The model under review builds one solid part; all positions refer to its coordinate system, in mm. A direction names the side the tool comes from. Round coordinates to 2 decimals unless told otherwise and drop trailing zeros. Order: outer loops, then holes, each group sorted by start corner. A loop starts at its lowest first (then second) coordinate and runs counter-clockwise, first axis right, second up.
```python
from build123d import *

# Parameters (mm, degrees)
SKETCH1_W           = 96.799999948
SKETCH1_H           = 98
BOSS_EXTRUDE1_DEPTH = 1.2192
CUT_EXTRUDE1_REACH  = 139.752
SKETCH5_R           = 1.0922
CUT_EXTRUDE2_REACH  = 139.752
SKETCH6_R           = 1.143
SKETCH10_W          = 5
SKETCH10_H          = 5.08
SKETCH10_R          = 1.143
BOSS_EXTRUDE2_DEPTH = 96.774
SKETCH13_W          = 86.614
SKETCH13_H          = 5
CUT_EXTRUDE3_DEPTH  = 5.08
BOSS_EXTRUDE3_DEPTH = 5.08
BOSS_EXTRUDE5_DEPTH = 5.08
BOSS_EXTRUDE6_DEPTH = 5.08
BOSS_EXTRUDE7_DEPTH = 5.08
BOSS_EXTRUDE8_DEPTH = 5.08


with BuildPart() as part:
    # Sketch1 → Boss-Extrude1 (new body)
    with BuildSketch(Plane(origin=(0, 0, 0), x_dir=(1, 0, 0), z_dir=(0, 1, 0))):
        with Locations((48.399999974, -49)):
            Rectangle(SKETCH1_W, SKETCH1_H)
    extrude(amount=BOSS_EXTRUDE1_DEPTH)

    # Sketch5 → Cut-Extrude1 (cut, up to next)
    with BuildSketch(Plane(origin=(0, 0, 0), x_dir=(-1, 0, 0), z_dir=(0, -1, 0)), mode=Mode.PRIVATE) as cut_extrude1_sk1:
        with Locations(Location((-3.5, -94.5, 0), (0, 0, 90))):
            Circle(SKETCH5_R)
    cut_extrude1_tool1 = extrude(cut_extrude1_sk1.sketch, amount=-CUT_EXTRUDE1_REACH, mode=Mode.PRIVATE) & part.part
    # Sketch5 → Cut-Extrude1 (cut, up to next)
    with BuildSketch(Plane(origin=(0, 0, 0), x_dir=(-1, 0, 0), z_dir=(0, -1, 0)), mode=Mode.PRIVATE) as cut_extrude1_sk2:
        with Locations(Location((-7.7, -95.3, 0), (0, 0, 90))):
            Circle(SKETCH5_R)
    cut_extrude1_tool2 = extrude(cut_extrude1_sk2.sketch, amount=-CUT_EXTRUDE1_REACH, mode=Mode.PRIVATE) & part.part
    # Sketch5 → Cut-Extrude1 (cut, up to next)
    with BuildSketch(Plane(origin=(0, 0, 0), x_dir=(-1, 0, 0), z_dir=(0, -1, 0)), mode=Mode.PRIVATE) as cut_extrude1_sk3:
        with Locations(Location((-21.3, -95.3, 0), (0, 0, 90))):
            Circle(SKETCH5_R)
    cut_extrude1_tool3 = extrude(cut_extrude1_sk3.sketch, amount=-CUT_EXTRUDE1_REACH, mode=Mode.PRIVATE) & part.part
    # Sketch5 → Cut-Extrude1 (cut, up to next)
    with BuildSketch(Plane(origin=(0, 0, 0), x_dir=(-1, 0, 0), z_dir=(0, -1, 0)), mode=Mode.PRIVATE) as cut_extrude1_sk4:
        with Locations(Location((-93.3, -94.5, 0), (0, 0, 90))):
            Circle(SKETCH5_R)
    cut_extrude1_tool4 = extrude(cut_extrude1_sk4.sketch, amount=-CUT_EXTRUDE1_REACH, mode=Mode.PRIVATE) & part.part
    # Sketch5 → Cut-Extrude1 (cut, up to next)
    with BuildSketch(Plane(origin=(0, 0, 0), x_dir=(-1, 0, 0), z_dir=(0, -1, 0)), mode=Mode.PRIVATE) as cut_extrude1_sk5:
        with Locations(Location((-93.3, -16.5, 0), (0, 0, 90))):
            Circle(SKETCH5_R)
    cut_extrude1_tool5 = extrude(cut_extrude1_sk5.sketch, amount=-CUT_EXTRUDE1_REACH, mode=Mode.PRIVATE) & part.part
    # Sketch5 → Cut-Extrude1 (cut, up to next)
    with BuildSketch(Plane(origin=(0, 0, 0), x_dir=(-1, 0, 0), z_dir=(0, -1, 0)), mode=Mode.PRIVATE) as cut_extrude1_sk6:
        with Locations(Location((-3.5, -16.5, 0), (0, 0, 90))):
            Circle(SKETCH5_R)
    cut_extrude1_tool6 = extrude(cut_extrude1_sk6.sketch, amount=-CUT_EXTRUDE1_REACH, mode=Mode.PRIVATE) & part.part
    # Sketch5 → Cut-Extrude1 (cut, up to next)
    with BuildSketch(Plane(origin=(0, 0, 0), x_dir=(-1, 0, 0), z_dir=(0, -1, 0)), mode=Mode.PRIVATE) as cut_extrude1_sk7:
        with Locations(Location((-7.7, -15.7, 0), (0, 0, 90))):
            Circle(SKETCH5_R)
    cut_extrude1_tool7 = extrude(cut_extrude1_sk7.sketch, amount=-CUT_EXTRUDE1_REACH, mode=Mode.PRIVATE) & part.part
    # Sketch5 → Cut-Extrude1 (cut, up to next)
    with BuildSketch(Plane(origin=(0, 0, 0), x_dir=(-1, 0, 0), z_dir=(0, -1, 0)), mode=Mode.PRIVATE) as cut_extrude1_sk8:
        with Locations(Location((-21.3, -15.7, 0), (0, 0, 90))):
            Circle(SKETCH5_R)
    cut_extrude1_tool8 = extrude(cut_extrude1_sk8.sketch, amount=-CUT_EXTRUDE1_REACH, mode=Mode.PRIVATE) & part.part
    add(cut_extrude1_tool1.solids().sort_by_distance((3.5, 0, 94.5))[0], mode=Mode.SUBTRACT)
    add(cut_extrude1_tool2.solids().sort_by_distance((7.7, 0, 95.3))[0], mode=Mode.SUBTRACT)
    add(cut_extrude1_tool3.solids().sort_by_distance((21.3, 0, 95.3))[0], mode=Mode.SUBTRACT)
    add(cut_extrude1_tool4.solids().sort_by_distance((93.3, 0, 94.5))[0], mode=Mode.SUBTRACT)
    add(cut_extrude1_tool5.solids().sort_by_distance((93.3, 0, 16.5))[0], mode=Mode.SUBTRACT)
    add(cut_extrude1_tool6.solids().sort_by_distance((3.5, 0, 16.5))[0], mode=Mode.SUBTRACT)
    add(cut_extrude1_tool7.solids().sort_by_distance((7.7, 0, 15.7))[0], mode=Mode.SUBTRACT)
    add(cut_extrude1_tool8.solids().sort_by_distance((21.3, 0, 15.7))[0], mode=Mode.SUBTRACT)

    # Sketch6 → Cut-Extrude2 (cut, up to next)
    with BuildSketch(Plane(origin=(0, 1.2192, 0), x_dir=(1, 0, 0), z_dir=(0, 1, 0)), mode=Mode.PRIVATE) as cut_extrude2_sk1:
        with Locations(Location((56.337499948, -7.540625, 0), (0, 0, 270))):
            Circle(SKETCH6_R)
    cut_extrude2_tool1 = extrude(cut_extrude2_sk1.sketch, amount=-CUT_EXTRUDE2_REACH, mode=Mode.PRIVATE) & part.part
    # Sketch6 → Cut-Extrude2 (cut, up to next)
    with BuildSketch(Plane(origin=(0, 1.2192, 0), x_dir=(1, 0, 0), z_dir=(0, 1, 0)), mode=Mode.PRIVATE) as cut_extrude2_sk2:
        with Locations(Location((40.462499948, -7.540625, 0), (0, 0, 270))):
            Circle(SKETCH6_R)
    cut_extrude2_tool2 = extrude(cut_extrude2_sk2.sketch, amount=-CUT_EXTRUDE2_REACH, mode=Mode.PRIVATE) & part.part
    # Sketch6 → Cut-Extrude2 (cut, up to next)
    with BuildSketch(Plane(origin=(0, 1.2192, 0), x_dir=(1, 0, 0), z_dir=(0, 1, 0)), mode=Mode.PRIVATE) as cut_extrude2_sk3:
        with Locations(Location((40.462499948, -90.459375, 0), (0, 0, 270))):
            Circle(SKETCH6_R)
    cut_extrude2_tool3 = extrude(cut_extrude2_sk3.sketch, amount=-CUT_EXTRUDE2_REACH, mode=Mode.PRIVATE) & part.part
    # Sketch6 → Cut-Extrude2 (cut, up to next)
    with BuildSketch(Plane(origin=(0, 1.2192, 0), x_dir=(1, 0, 0), z_dir=(0, 1, 0)), mode=Mode.PRIVATE) as cut_extrude2_sk4:
        with Locations(Location((56.337499948, -90.459375, 0), (0, 0, 270))):
            Circle(SKETCH6_R)
    cut_extrude2_tool4 = extrude(cut_extrude2_sk4.sketch, amount=-CUT_EXTRUDE2_REACH, mode=Mode.PRIVATE) & part.part
    add(cut_extrude2_tool1.solids().sort_by_distance((56.3375, 1.2192, 7.540625))[0], mode=Mode.SUBTRACT)
    add(cut_extrude2_tool2.solids().sort_by_distance((40.4625, 1.2192, 7.540625))[0], mode=Mode.SUBTRACT)
    add(cut_extrude2_tool3.solids().sort_by_distance((40.4625, 1.2192, 90.459375))[0], mode=Mode.SUBTRACT)
    add(cut_extrude2_tool4.solids().sort_by_distance((56.3375, 1.2192, 90.459375))[0], mode=Mode.SUBTRACT)

    # Sketch10 → Boss-Extrude2 (add)
    with BuildSketch(Plane(origin=(96.799999948, 0, 0), x_dir=(0, 0, -1), z_dir=(1, 0, 0))):
        with Locations((-49, 3.7592)):
            Rectangle(SKETCH10_W, SKETCH10_H)
        with Locations((-49, 2.64795)):
            Circle(SKETCH10_R, mode=Mode.SUBTRACT)
    extrude(amount=-BOSS_EXTRUDE2_DEPTH)

    # Sketch13 → Cut-Extrude3 (cut)
    with BuildSketch(Plane(origin=(0, 6.2992, 0), x_dir=(1, 0, 0), z_dir=(0, 1, 0))):
        with Locations((48.412999948, -49)):
            Rectangle(SKETCH13_W, SKETCH13_H)
    extrude(amount=-CUT_EXTRUDE3_DEPTH, mode=Mode.SUBTRACT)

    # Sketch14 → Boss-Extrude3 (add)
    with BuildSketch(Plane.XZ):
        Polygon((0, 49), (0, 51.54), (5.08, 51.54), (5.08, 46.46), (0, 46.46), align=None)
        Polygon((96.799999948, 49), (96.799999948, 51.54), (91.719999948, 51.54), (91.719999948, 46.46), (96.799999948, 46.46), align=None)
    extrude(amount=BOSS_EXTRUDE3_DEPTH)

    # Sketch15 → Boss-Extrude5 (add)
    with BuildSketch(Plane.ZY):
        Polygon((51.54, -5.08), (46.46, -5.08), (46.46, -5.479804671), align=None)
    extrude(amount=-BOSS_EXTRUDE5_DEPTH)

    # Sketch16 → Boss-Extrude6 (add)
    with BuildSketch(Plane(origin=(96.799999948, 0, 0), x_dir=(0, 0, -1), z_dir=(1, 0, 0))):
        Polygon((-46.46, -5.08), (-51.54, -5.08), (-46.46, -5.479804671), align=None)
    extrude(amount=-BOSS_EXTRUDE6_DEPTH)

    # Sketch17 → Boss-Extrude7 (add)
    with BuildSketch(Plane(origin=(96.799999948, 0, 0), x_dir=(0, 0, -1), z_dir=(1, 0, 0))):
        Polygon((-46.5, 6.2992), (-51.5, 6.2992), (-51.5, 6.692708534), align=None)
    extrude(amount=-BOSS_EXTRUDE7_DEPTH)

    # Sketch18 → Boss-Extrude8 (add)
    with BuildSketch(Plane.ZY.offset(-0.025999948)):
        Polygon((46.5, 6.2992), (51.5, 6.2992), (51.5, 6.692708534), align=None)
    extrude(amount=-BOSS_EXTRUDE8_DEPTH)


solid = part.part
```
(1) Consider section A-A (y = -2). Write out the cut boundary in (x, z), and give its area (3 significant figures).
Data:
outline: (0, 46.46) - (5.08, 46.46) - (5.08, 51.54) - (0, 51.54) - close; (91.72, 46.46) - (96.8, 46.46) - (96.8, 51.54) - (91.72, 51.54) - close
area: 51.6 mm2
(2) To check wall thickness, follow probe 1 along Z at (x, y) = (93.3, 0.7); probe 2 along X at (y, z) = (0.9, 94.5); probe 3 along Y at (x, z) = (58, 84). State the ranges of each line that lie inside material, in increasing order.
Data:
probe 1: z = 0 to 15.41, 17.59 to 93.41, 95.59 to 98
probe 2: x = 0 to 2.41, 4.59 to 6.96, 8.44 to 20.56, 22.04 to 92.21, 94.39 to 96.8
probe 3: y = 0 to 1.22
(3) Insertion check: pin 1 (1.7 mm diameter, centred on x = 3.5, z = 16.5, fed in from -Y); pin 2 (1.5 mm diameter, centred on x = 2.5, y = 3.5, fed in from +Z); pin 3 (3 mm diameter, centred on x = 40.46, z = 90.46, fed in from -Y); pin 4 (4 mm diameter, centred on x = 93, y = -3, fed in from -Z). Each pin has a flat end and moves straight along its axis. Give the tip position at first contact, or say it passes through.
Data:
pin 1: passes through
pin 2: stops at z = 51.5
pin 3: stops at y = 0
pin 4: stops at z = 46.46
(4) For faces 1 (the flat face through (5.106, 4, 49)), 2 (the flat face through (94, -3, 46.46)), 3 (the flat face through (94, -3, 51.54)), 4 (the flat face through (3, 4, 46.5)), 5 (the flat face through (94, 4, 51.5)), list the 3-axis set-ups (+Z, -Z, +X, -X, +Y, -Y) from which the entire face can be reached by the end or side of a thin tool; tool diameter is ignored.
Data:
face 1: +Z, -Z, +Y
face 2: -Z, +X, -X, -Y
face 3: +Z, +X, -X, -Y
face 4: -Z, +X, -X, +Y
face 5: +Z, +X, -X, +Y
(5) Consider section B-B (x = 15). Write out the cut boundary in (y, z).
Data:
outline: (0, 0) - (1.22, 0) - (1.22, 98) - (0, 98) - close
(6) Consider section C-C (z = 76). Write out the cut boundary in (x, y), and give its area (3 significant figures).
Data:
outline: (0, 0) - (96.8, 0) - (96.8, 1.22) - (0, 1.22) - close
area: 118 mm2
(7) Draft analysis for pull direction X (two halves, no side actions). For faces 6 (the cylindrical face through (2.602, 3.42, 49.842)), 7 (the cylindrical face through (21.35, 0.6, 96.39)), 8 (the flat face through (0, 0, 49)), state which applies: pulls with the +X half, pulls with the -X half, needs draft (parallel to the pull), parting line crosses it, or undercut.
Data:
face 6: needs draft
face 7: undercut
face 8: pulls with the -X half
